```python
from build123d import *

# Parameters (mm, degrees)
F0_W     = 50.8
F0_H     = 101.6
F1_DEPTH = 44.45
F2_W     = 50.8
F2_H     = 101.6
F3_DEPTH = 12.7
F4_W     = 50.8
F4_H     = 101.6
F5_DEPTH = 12.7
F6_W     = 2082.8
F6_H     = 19.05
F7_DEPTH = 12.7
F8_W     = 12.7
F8_H     = 25.4
F9_DEPTH = 31.751


with BuildPart() as f1:
    # F0 (on Top) → F1 (new body)
    with BuildSketch(Plane.XY):
        Polygon((1020.749743, -440.41436), (-960.450257, -440.41436), (-960.450257, -542.01436), (-960.450257, -592.81436), (1020.749743, -592.81436), (1020.749743, -542.01436), align=None)
        with Locations((-985.850257, -491.21436)):
            Rectangle(F0_W, F0_H)
        with Locations((1046.149743, -491.21436)):
            Rectangle(F0_W, F0_H)
    extrude(amount=F1_DEPTH)

    # F2 (on Top) → F3 (cut)
    with BuildSketch(Plane.XY):
        with Locations((-985.850257, -491.21436)):
            Rectangle(F2_W, F2_H)
        with Locations((1046.149743, -491.21436)):
            Rectangle(F2_W, F2_H)
    extrude(amount=F3_DEPTH, mode=Mode.SUBTRACT)

    # F4 (on face) → F5 (cut)
    with BuildSketch(Plane.XY.offset(44.45)):
        with Locations((1046.149743, -491.21436)):
            Rectangle(F4_W, F4_H)
        with Locations((-985.850257, -491.21436)):
            Rectangle(F4_W, F4_H)
    extrude(amount=-F5_DEPTH, mode=Mode.SUBTRACT)

    # F6 (on face) → F7 (cut)
    with BuildSketch(Plane(origin=(0, -440.41436, 0), x_dir=(-1, 0, 0), z_dir=(0, 1, 0))):
        with Locations((-30.149743, 22.225)):
            Rectangle(F6_W, F6_H)
    extrude(amount=-F7_DEPTH, mode=Mode.SUBTRACT)

    # F8 (on face) → F9 (cut, through all)
    with BuildSketch(Plane(origin=(0, 0, 12.7), x_dir=(1, 0, 0), z_dir=(0, 0, -1))):
        with Locations((-985.850257, 497.56436)):
            Rectangle(F8_W, F8_H)
        with Locations((1046.149743, 497.56436)):
            Rectangle(F8_W, F8_H)
    extrude(amount=-F9_DEPTH, mode=Mode.SUBTRACT)


solid = f1.part
```
Part model, mm, in its own coordinate system. A direction names the side the tool comes from. Round coordinates to 2 decimals unless told otherwise and drop trailing zeros. Loops run counter-clockwise (first coordinate to the right, second up) from the corner with the lowest first, then second, coordinate; pieces in that order, holes last.
1. Slice it at B-B (z = 24.5). Give the cut face in (x, y).
Solutions:
outline: (-1011.25, -542.01) - (-960.45, -542.01) - (-960.45, -592.81) - (1020.75, -592.81) - (1020.75, -542.01) - (1071.55, -542.01) - (1071.55, -453.11) - (-1011.25, -453.11) - close; hole (-992.2, -510.26) - (-979.5, -510.26) - (-979.5, -484.86) - (-992.2, -484.86) - close; hole (1039.8, -510.26) - (1052.5, -510.26) - (1052.5, -484.86) - (1039.8, -484.86) - close
2. Flat gauge pins, fed straight in: pin 1 (12 mm diameter, centred on y = -577.5, z = 25.5, fed in from +X); pin 2 (1.5 mm diameter, centred on x = -272, z = 17, fed in from +Y); pin 3 (9.5 mm diameter, centred on x = 1044.5, z = 22.5, fed in from -Y). Where does each tip first touch, or does it go through?
Solutions:
pin 1: stops at x = 1020.75
pin 2: stops at y = -453.11
pin 3: stops at y = -542.01
3. Slice it at A-A (x = -482). Give the cut face in (y, z).
Solutions:
outline: (-592.81, 0) - (-440.41, 0) - (-440.41, 12.7) - (-453.11, 12.7) - (-453.11, 31.75) - (-440.41, 31.75) - (-440.41, 44.45) - (-592.81, 44.45) - close
4. Slice it at C-C (y = -570). Give the cut face in (x, z), and give its area (3 significant figures).
Solutions:
outline: (-960.45, 0) - (1020.75, 0) - (1020.75, 44.45) - (-960.45, 44.45) - close
area: 88,100 mm2
5. 3-axis set-ups, long thin cutter, end or side, ignore diameter. For faces 1 (the face through (-997, -497, 12.7)), 2 (the face through (1035, -497, 12.7)), 3 (the face through (1035, -497, 31.75)): which of +Z, -Z, +X, -X, +Y, -Y reach the whole face in a straight line?
Solutions:
face 1: -Z, -X, +Y, -Y
face 2: -Z, +X, +Y, -Y
face 3: +Z, +X, +Y, -Y
6. Drill centre lines: line 1 along Y through (x, z) = (242, 22.5); line 2 along Z through (x, y) = (189.5, -447); line 3 along X through (y, z) = (-454.5, 40.5). Where is each one in solid material? Low to high.
Solutions:
line 1: y = -592.81 to -453.11
line 2: z = 0 to 12.7, 31.75 to 44.45
line 3: x = -960.45 to 1020.75
